Build history of the part. All positions in model axes, mm. Give positions to 0.01 mm unless a question says otherwise; leave off trailing zeros. Write each loop counter-clockwise with the first axis right and the second up, starting at its lowest first coordinate (ties: lowest second). Pieces come first, ordered by that corner, then holes.
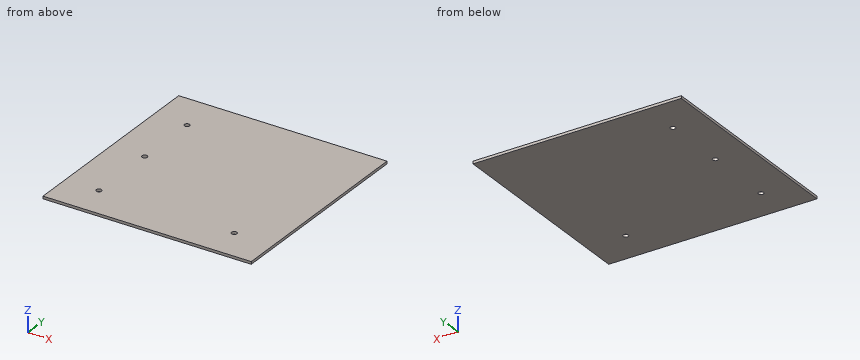
from build123d import *

# Parameters (mm, degrees)
F0_R     = 5
F0_W     = 260
F0_H     = 130
F1_DEPTH = 5
F0_W_2   = 130
F0_H_2   = 120
F2_DEPTH = 5


with BuildPart() as f1:
    # F0 (on Top) → F1 (new body)
    with BuildSketch(Plane.XY):
        Polygon((200, 200), (-200, 200), (-200, 190), (60, 190), (60, 180), (190, 180), (190, 60), (190, -200), (200, -200), align=None)
        Polygon((60, 190), (-200, 190), (-200, 60), (60, 60), (60, 180), align=None)
        with Locations((-135, 125)):
            Circle(F0_R, mode=Mode.SUBTRACT)
        with Locations((-70, -5)):
            Rectangle(F0_W, F0_H)
        with Locations((-135, 0)):
            Circle(F0_R, mode=Mode.SUBTRACT)
        Polygon((60, -200), (190, -200), (190, 60), (60, 60), (60, -70), align=None)
        with Locations((125, -135)):
            Circle(F0_R, mode=Mode.SUBTRACT)
        with Locations((-70, -135)):
            Rectangle(F0_W, F0_H)
        with Locations((-135, -135)):
            Circle(F0_R, mode=Mode.SUBTRACT)
    extrude(amount=F1_DEPTH)

    # F0 (on Top) → F2 (join)
    with BuildSketch(Plane.XY):
        with Locations((125, 120)):
            Rectangle(F0_W_2, F0_H_2)
    extrude(amount=F2_DEPTH)


solid = f1.part
1. Saw through at D-D on y = -135. Give the cut face in (x, z).
2. Drill centre lines: line 1 along Y through (x, z) = (-135, 3.35); line 2 along Y through (x, z) = (123, 2.4); line 3 along X through (y, z) = (3, 0.4). Where is each one in solid material? Low to high.
3. Saw through at A-A on y = 0. Give the cut face in (x, z).
4. Saw through at B-B on x = -135. Give the cut face in (y, z).
5. Drop a flat-ended pin along its axis: pin 1 (12 mm diameter, centred on x = -120.5, y = -65, fed in from -Z). Give the stop position or say it passes through.
Outcome:
1. outline: (-200, 0) - (-140, 0) - (-140, 5) - (-200, 5) - close; (-130, 0) - (120, 0) - (120, 5) - (-130, 5) - close; (130, 0) - (200, 0) - (200, 5) - (130, 5) - close
2. line 1: y = -200 to -140, -130 to -5, 5 to 120, 130 to 200
2. line 2: y = -200 to -139.58, -130.42 to 200
2. line 3: x = -200 to -139, -131 to 200
3. outline: (-200, 0) - (-140, 0) - (-140, 5) - (-200, 5) - close; (-130, 0) - (200, 0) - (200, 5) - (-130, 5) - close
4. outline: (-200, 0) - (-140, 0) - (-140, 5) - (-200, 5) - close; (-130, 0) - (-5, 0) - (-5, 5) - (-130, 5) - close; (5, 0) - (120, 0) - (120, 5) - (5, 5) - close; (130, 0) - (200, 0) - (200, 5) - (130, 5) - close
5. pin 1: stops at z = 0
